from build123d import *


with BuildPart() as part:
    # Sketch1 → Base-Revolve (revolve)
    with BuildSketch(Plane.XY):
        with BuildLine():
            Line((-177, 35), (-177, 46.5))
            ThreePointArc((-177, 46.5), (-176.707106781, 47.207106781), (-176, 47.5))
            Line((-176, 47.5), (176, 47.5))
            ThreePointArc((176, 47.5), (176.707106781, 47.207106781), (177, 46.5))
            Line((177, 46.5), (177, 35))
            Line((177, 35), (110.962610506, 35))
            Line((110.962610506, 35), (109, 36))
            Line((109, 36), (107, 36))
            Line((107, 36), (107, 34))
            Line((107, 34), (97.176326981, 34))
            ThreePointArc((97.176326981, 34), (97.002678803, 34.015192247), (96.834306837, 34.060307379))
            Line((96.834306837, 34.060307379), (87.549522195, 37.439692621))
            ThreePointArc((87.549522195, 37.439692621), (87.381150229, 37.484807753), (87.207502051, 37.5))
            Line((87.207502051, 37.5), (-87.207502051, 37.5))
            ThreePointArc((-87.207502051, 37.5), (-87.381150229, 37.484807753), (-87.549522195, 37.439692621))
            Line((-87.549522195, 37.439692621), (-96.834306837, 34.060307379))
            ThreePointArc((-96.834306837, 34.060307379), (-97.002678803, 34.015192247), (-97.176326981, 34))
            Line((-97.176326981, 34), (-107, 34))
            Line((-107, 34), (-107, 36))
            Line((-107, 36), (-109, 36))
            Line((-109, 36), (-110.962610506, 35))
            Line((-110.962610506, 35), (-177, 35))
        make_face()
    revolve(axis=Axis((-177, 0, 0), (1, 0, 0)))

    # Sketch5 → Reifning 2.5 x 30 gr (revolve, cut)
    with BuildSketch(Plane.XY):
        Polygon((-177, 35), (-177, 35.866025404), (-175.5, 35), align=None)
        Polygon((177, 35), (175.5, 35), (177, 35.866025404), align=None)
    revolve(axis=Axis((0, 0, 0), (1, 0, 0)), mode=Mode.SUBTRACT)


solid = part.part
Build history of the part. All positions in model axes, mm. A direction names the side the tool comes from. Coordinates: 2 decimals unless noted, no trailing zeros. Write each loop counter-clockwise with the first axis right and the second up, starting at its lowest first coordinate (ties: lowest second). Pieces come first, ordered by that corner, then holes. Notation, with made-up numbers: (2, 3.5) -> (53, 3.5) arc R32 ccw to (53, 36.5) -> close; hole circle Ø6 at (75, 25). An arc over 180 degrees is marked (long way). Use CSV: the item, a comma, the result in double quotes. Start each with the question number.
Q1. Drill centre lines: probe 1 along Z at (x, y) = (150, 0); probe 2 along Z at (x, y) = (22.5, 0); probe 3 along Y at (x, z) = (-109, 23). Where is each one in solid material? Low to high.
Q2. Cut at A-A, the plane x = 147. List the corners of the cut face in (y, z), then the cut area to 3 significant figures.
Q3. Flat gauge pins, fed straight in: pin 1 Ø3 at (x, y) = (-40, 35.5) entering from +Z; pin 2 Ø2 at (x, z) = (29, -17.5) entering from -Y; pin 3 Ø6 at (x, z) = (42.5, 14.5) entering from -Y; pin 4 Ø2 at (y, z) = (26, -17) entering from -X. Where does each tip first touch, or does it go through?
Q4. 3-axis set-ups, long thin cutter, end or side, ignore diameter. For faces 1 (the cylindrical face through (102.02, 18.28, 28.67)), 2 (the flat face through (107, 32, -13)), 3 (the cylindrical face through (-144, -28, -21)), 4 (the cylindrical face through (143, -28, -21)), 5 (the flat face through (177, 24, -27)): which of +Z, -Z, +X, -X, +Y, -Y reach the whole face in a straight line?
Q5. Pull direction Y, two halves, no side cores. Call faces 6 (the cylindrical face through (2.46, -10.3, -46.37)), 7 (the cylindrical face through (-108.014, -4.686, 35.694)), 8 (the flat face through (-177, -24, -27)): released by +Y, released by -Y, zero draft, split by the parting line, or undercut.
Q6. Cut at B-B, the plane x = 65. List the corners of the cut face in (y, z), then the cut area to 3 significant figures.
Checked values:
1,probe 1,"z = -47.5 to -35, 35 to 47.5"
1,probe 2,"z = -47.5 to -37.5, 37.5 to 47.5"
1,probe 3,"y = -41.56 to -27.69, 27.69 to 41.56"
2,outline,"circle Ø95 at (0, 0); hole circle Ø70 at (0, 0)"
2,area,"3,240 mm²"
3,pin 1,"stops at z = 33.17"
3,pin 2,"stops at y = -44.54"
3,pin 3,"stops at y = -46.09"
3,pin 4,"passes through"
4,face 1,"+X, -X"
4,face 2,"none"
4,face 3,"-X"
4,face 4,"+X"
4,face 5,"+Z, -Z, +X, +Y, -Y"
5,face 6,"split by the parting line"
5,face 7,"undercut"
5,face 8,"zero draft"
6,outline,"circle Ø95 at (0, 0); hole circle Ø75 at (0, 0)"
6,area,"2,670 mm²"
